from build123d import *

# Parameters (mm, degrees)
BOSS_EXTRUDE1_DEPTH = 11.1125
BOSS_EXTRUDE2_START = 11.1125
SKETCH1_4_R         = 12.7
BOSS_EXTRUDE2_DEPTH = 19.05
BOSS_EXTRUDE4_START = -11.1125
SKETCH1_6_R         = 22.225
SKETCH1_6_R_2       = 12.7
BOSS_EXTRUDE4_DEPTH = 19.05


with BuildPart() as part:
    # Sketch1 → Boss-Extrude1 (new, symmetric)
    with BuildSketch(Plane.XY):
        with BuildLine():
            Line((28.443390267, 0), (41.275, -22.225))
            Line((41.275, -22.225), (187.325, -22.225))
            Line((187.325, -22.225), (187.325, -2.54))
            ThreePointArc((187.325, -2.54), (186.581051224, -0.743948776), (184.785, 0))
            Line((184.785, 0), (28.443390267, 0))
        make_face()
    extrude(amount=BOSS_EXTRUDE1_DEPTH, both=True)

    # Sketch1<4> → Boss-Extrude2 (add)
    with BuildSketch(Plane.XY.offset(BOSS_EXTRUDE2_START)):
        with BuildLine():
            ThreePointArc((25.200781238, 0), (23.100716135, 0.79375), (22.050683583, 2.778125))
            ThreePointArc((22.050683583, 2.778125), (-16.66875, 14.700455722), (0, -22.225))
            Line((0, -22.225), (85.725, -22.225))
            Line((85.725, -22.225), (79.769829198, 0))
            Line((79.769829198, 0), (25.200781238, 0))
        make_face()
        with Locations(Location((0, 0, 0), (0, 0, 180))):
            Circle(SKETCH1_4_R, mode=Mode.SUBTRACT)
        with BuildLine():
            Line((111.125, 0), (111.125, -22.225))
            Line((111.125, -22.225), (187.325, -22.225))
            Line((187.325, -22.225), (187.325, -2.54))
            ThreePointArc((187.325, -2.54), (186.581051224, -0.743948776), (184.785, 0))
            Line((184.785, 0), (158.75, 0))
            Line((158.75, 0), (158.75, 28.575))
            ThreePointArc((158.75, 28.575), (156.890128061, 33.065128061), (152.4, 34.925))
            Line((152.4, 34.925), (139.7, 34.925))
            ThreePointArc((139.7, 34.925), (129.503262126, 14.115512806), (111.125, 0))
        make_face()
    extrude(amount=BOSS_EXTRUDE2_DEPTH)

    # Sketch1<6> → Boss-Extrude4 (add)
    with BuildSketch(Plane.XY.offset(BOSS_EXTRUDE4_START)):
        Circle(SKETCH1_6_R)
        with Locations(Location((0, 0, 0), (0, 0, 180))):
            Circle(SKETCH1_6_R_2, mode=Mode.SUBTRACT)
        with BuildLine():
            ThreePointArc((22.225, 0), (15.715448212, -15.715448212), (0, -22.225))
            Line((0, -22.225), (41.275, -22.225))
            Line((41.275, -22.225), (28.443390267, 0))
            Line((28.443390267, 0), (25.200781238, 0))
            ThreePointArc((25.200781238, 0), (23.100716135, 0.79375), (22.050683583, 2.778125))
            ThreePointArc((22.050683583, 2.778125), (22.181378087, 1.391794231), (22.225, 0))
        make_face()
        Polygon((28.443390267, 0), (41.275, -22.225), (85.725, -22.225), (79.769829198, 0), align=None)
        with BuildLine():
            Line((187.325, -22.225), (187.325, -2.54))
            ThreePointArc((187.325, -2.54), (186.581051224, -0.743948776), (184.785, 0))
            Line((184.785, 0), (158.75, 0))
            Line((158.75, 0), (111.125, 0))
            Line((111.125, 0), (111.125, -22.225))
            Line((111.125, -22.225), (187.325, -22.225))
        make_face()
        Polygon((85.725, -22.225), (79.769829198, 0), (111.125, 0), (111.125, -22.225), align=None)
    extrude(amount=-BOSS_EXTRUDE4_DEPTH)


solid = part.part
Geometry check sheet. Reference: the model listing, model coordinates, mm. A direction names the side the tool comes from. Round coordinates to 2 decimals unless told otherwise and drop trailing zeros. Order: outer loops, then holes, each group sorted by start corner. A loop starts at its lowest first (then second) coordinate and runs counter-clockwise, first axis right, second up. Notation, with made-up numbers: M 33.5,-23.75 L 38.5,-23.75 A17 ccw 38.5,4.25 Z; hole C -28.75,34.5 d8. An arc over 180 degrees is marked long. Answer in a Markdown table with one row per item. Add a question column.
Item 1: Sectioned sample at A-A, the plane z = 15. Enter the section's corners in (x, y) (3 decimals).
Item 2: Set-up check for faces 1 (the face through (34.77, -10.96, 0.16)), 2 (the face through (145, 14, 11.112)), 3 (the face through (129.71, 14.37, 20.5)), 4 (the face through (111.125, -11, 21)): record each of +Z, -Z, +X, -X, +Y, -Y from which the full face is reachable in a straight line by a thin tool's end or side.
Item 3: Draft check along X on faces 5 (the face through (146, 34.925, 21)), 6 (the face through (187.325, -13, 0)), 7 (the face through (-5.86, 11.267, 20.504)). Enter one of: released by +X, released by -X, zero draft, split by the parting line, or undercut.
Item 4: Depth check by flat-ended pin: pin 1 Ø2 at (y, z) = (-4.5, -22) entering from -X; pin 2 Ø1.5 at (y, z) = (5, 17.5) entering from -X; pin 3 Ø2 at (x, z) = (62.5, 11.5) entering from +Y. Enter the tip coordinate at first touch or a pass-through.
Item 5: Sectioned sample at C-C, the plane x = 4. Enter the section's corners in (y, z) (1 decimal), plus the area to 3 significant figures.
Item 6: Material ranges on L1, parallel to Z at x = 0, y = 15; L2, parallel to Y at x = 0, z = 17.25 (3 decimals); L3, parallel to X at y = 1.5, z = 19, recorded low to high. Write a range as [from, to].
Item 7: Sectioned sample at D-D, the plane z = -19. Enter the section's corners in (x, y) (3 decimals).
Item 8: Sectioned sample at B-B, the plane y = 18.5. Enter the section's corners in (x, z).
Filled in:
| question | item | result |
|---|---|---|
| 1 | outline | M 0,-22.225 L 85.725,-22.225 L 79.77,0 L 25.201,0 A3.175 cw 22.051,2.778 A22.225 ccw long Z; M 111.125,-22.225 L 187.325,-22.225 L 187.325,-2.54 A2.54 ccw 184.785,0 L 158.75,0 L 158.75,28.575 A6.35 ccw 152.4,34.925 L 139.7,34.925 A50.8 cw 111.125,0 Z; hole C 0,0 d25.4 |
| 2 | face 1 | -X, -Y |
| 2 | face 2 | -Z, +X, -X, +Y |
| 2 | face 3 | +Z, -Z, +Y |
| 2 | face 4 | +Z, +Y, -Y |
| 3 | face 5 | zero draft |
| 3 | face 6 | released by +X |
| 3 | face 7 | undercut |
| 4 | pin 1 | stops at x = -21.95 |
| 4 | pin 2 | stops at x = -21.81 |
| 4 | pin 3 | stops at y = 0 |
| 5 | outline | M -22.2,-30.2 L -12.1,-30.2 L -12.1,-11.1 L -22.2,-11.1 Z; M -22.2,11.1 L -12.1,11.1 L -12.1,30.2 L -22.2,30.2 Z; M 12.1,-30.2 L 21.9,-30.2 L 21.9,-11.1 L 12.1,-11.1 Z; M 12.1,11.1 L 21.9,11.1 L 21.9,30.2 L 12.1,30.2 Z |
| 5 | area | 761 mm² |
| 6 | L1 | z = [-30.16, -11.11], [11.11, 30.16] |
| 6 | L2 | y = [-22.225, -12.7], [12.7, 22.225] |
| 6 | L3 | x = [-22.17, -12.61], [12.61, 22.5], [114.17, 158.75] |
| 7 | outline | M 0,-22.225 L 187.325,-22.225 L 187.325,-2.54 A2.54 ccw 184.785,0 L 25.201,0 A3.175 cw 22.051,2.778 A22.225 ccw long Z; hole C 0,0 d25.4 |
| 8 | outline | M -12.32,-30.16 L 12.32,-30.16 L 12.32,-11.11 L -12.32,-11.11 Z; M -12.32,11.11 L 12.32,11.11 L 12.32,30.16 L -12.32,30.16 Z; M 132.71,11.11 L 158.75,11.11 L 158.75,30.16 L 132.71,30.16 Z |
